Autodesk Inventor part; units mm, degrees
ref_plane "YZ Plane" through (0, 0, 0) normal (1, 0, 0) x (0, 1, 0)
ref_plane "XZ Plane" through (0, 0, 0) normal (0, 1, 0) x (-1, 0, 0)
ref_plane "XY Plane" through (0, 0, 0) normal (0, 0, 1) x (1, 0, 0)
sketch "Sketch1" plane through (0, 0, 0) normal (0, 1, 0) x (-1, 0, 0)
  circle A0 centre (0, 0) radius 3.05
  dimension "d0" = 6.1
extrude "Extrusion1" add sketch "Sketch1" along normal blind 4
sketch "Sketch2" plane through (0, 0, 0) normal (1, 0, 0) x (0, 1, 0)
  line L0 (12.1205, 0) -> (4, 0)
  line L1 (4, -3.05) -> (4, 3.05)
  arc A0 (10.3569, -1.4766) -> (12.1205, 0) centre (10.6205, 0) ccw
  line L2 (4, -0.9136) -> (10.6205, -1.5)
  line L3 (4, -0.9136) -> (4, 0)
  point P0 (0, 0)
  dimension "d3" = 3
revolve "Revolution1" add sketch "Sketch2" angle 360 about axis through (0, 12.1205, 0) along (0, -1, 0) contours A0 L2 L1 L0
sketch "Sketch3" plane through (0, 0, 0) normal (0, -1, 0) x (1, 0, 0)
  line L0 (6.5, 4) -> (-6.5, 4)
  line L1 (-6.5, 4) -> (-6.5, -4)
  line L2 (-6.5, -4) -> (6.5, -4)
  line L3 (6.5, -4) -> (6.5, 4)
  point P0 (0, 0)
  point P1 (-6.5, 0)
  point P2 (0, 4)
  dimension "d5" = 13
  dimension "d6" = 8
extrude "Extrusion2" add sketch "Sketch3" along normal blind 10
properties part number "toggle switch"
The listing builds one solid part. Answer for the finished solid, in the listing's coordinates (mm). A direction names the side the tool comes from. Give positions to 0.01 mm unless a question says otherwise; leave off trailing zeros. Write each loop counter-clockwise with the first axis right and the second up, starting at its lowest first coordinate (ties: lowest second). Pieces come first, ordered by that corner, then holes. Notation, with made-up numbers: (-6.75, -39) -> (25.25, -39) arc R13 ccw to (25.25, -21) -> close; hole circle Ø11 at (54, 24.5). An arc over 180 degrees is marked (long way). One line per question, with ' | ' between items. Start each with the question number.
1. Given pin 1 Ø3 at (x, z) = (1, 1) entering from +Y; pin 2 Ø4 at (x, z) = (-2.5, 1.5) entering from +Y; pin 3 Ø3 at (x, y) = (0, 6.5) entering from -Z; pin 4 Ø1.5 at (y, z) = (6.5, 2) entering from +X, each flat-ended and moving along its own axis, determine where each tip first touches the part or whether it passes through.
2. Section C-C (y = 10) is taken. Determine the outline of the cut face in (x, z), plus the area to 3 significant figures.
3. Section B-B (y = 3.5) is taken. Determine the outline of the cut face in (x, z).
4. Find the intervals of material crossed by probe 1 along Y at (x, z) = (-3.75, -1.25); probe 2 along Y at (x, z) = (1.75, -1); probe 3 along Z at (x, y) = (-2, 3), in increasing order.
5. For faces 1 (the flat face through (-1, 4, 1)), 2 (the cylindrical face through (3.047, 1.972, -0.134)), 3 (the flat face through (0, -5, 4)), determine the directions among +Z, -Z, +X, -X, +Y, -Y from which every point of the face is accessible in a straight line to the end or side of a thin tool.
6. Section A-A (x = 5.25) is taken. Determine the outline of the cut face in (y, z).
Response values:
1) pin 1: y = 12.12 | pin 2: y = 11.81 | pin 3: z = -1.27 | pin 4: through
2) outline: circle Ø2.89 at (0, 0) | area: 6.56 mm2
3) outline: circle Ø6.1 at (0, 0)
4) probe 1: -10 to 0 | probe 2: -10 to 4 | probe 3: -2.3 to 2.3
5) face 1: none | face 2: +Y | face 3: +Z, +X, -X, +Y, -Y
6) outline: (-10, -4) -> (0, -4) -> (0, 4) -> (-10, 4) -> close
